Solid Edge part; units mm, degrees
sketch "Sketch1" plane through (0, 0, 0) normal (0, -1, 0) x (1, 0, 0)
  line L0 (-30, 0) -> (-5, 0)
  line L1 (-5, 0) -> (-5, -160)
  line L2 (-5, -160) -> (-20, -160)
  line L3 (-20, -160) -> (-20, -10)
  line L4 (-20, -10) -> (-30, -10)
  line L5 (-30, -10) -> (-30, 0)
  dimension "D1" = 30
  dimension "D2" = 20
revolve "RevolvedProtrusion1" add sketch "Sketch1" angle 360 about axis through (0, 0, 54) along (0, 0, -1)
sketch "Sketch2" plane through (0, 0, -160) normal (0, 0, -1) x (0, 1, 0)
  circle A0 centre (0, 0) radius 10
  circle A1 centre (0, 0) radius 20
extrude "Cutout1" cut sketch "Sketch2" against normal blind 20
cosmetic_thread "Thread1"
sketch "Sketch3" plane through (0, 0, 0) normal (0, 0, 1) x (1, 0, 0)
  circle A0 centre (0, 0) radius 30
  circle A1 centre (0, 0) radius 5
extrude "Ausprägung_1" add sketch "Sketch3" along normal blind 30
sketch "Sketch4" plane through (0, 0, 0) normal (0, 0, 1) x (1, 0, 0)
  line L0 (-61, 50) -> (-11, 50)
  line L1 (-11, 50) -> (-11, -50)
  line L2 (-11, -50) -> (-61, -50)
  line L3 (-61, -50) -> (-61, 50)
extrude "Cutout2" cut sketch "Sketch4" along normal up to next
mirror "Mirror1" about plane through (0, 0, 0) normal (1, 0, 0) of "Cutout2"
hole "Bohrung_1" at (11, -20, 15) direction (-1, 0, 0) diameter 10 end through all
hole "Hole1" at (11, 20, 15) direction (-1, 0, 0) diameter 10 end through all
extrude "Cutout4" [suppressed]
chamfer "Fase_2" distance 1 angle 45 2 edges at (0, -20, -140) (0, -10, -160)
chamfer "Fase_3" distance 1 angle 45 2 edges at (-5, 0, 30) (5, 0, -160)
properties material "Stahl"
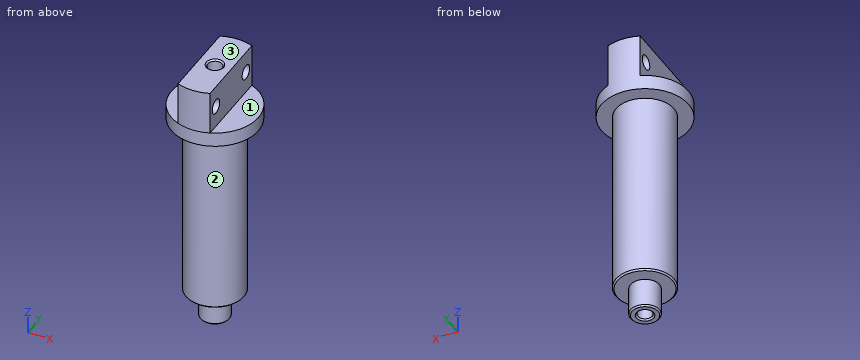
Could you check a few things on this model? Use its own coordinates, in mm. Face numbers are marked on the shaded views. A direction names the side the tool comes from. Give positions to 0.01 mm unless a question says otherwise; leave off trailing zeros. Loops run counter-clockwise (first coordinate to the right, second up) from the corner with the lowest first, then second, coordinate; pieces in that order, holes last. Notation, with made-up numbers: (78.25, 49) -> (93.25, 49) arc R20 ccw to (93.25, 53) -> close; hole circle Ø1 at (70.25, 71.25). An arc over 180 degrees is marked (long way). Return JSON: item names as keys, results as strings.
Item 1: If we section it at B-B on z = 15: List the corners of the cut face in (x, y) for me, plus the area to 3 significant figures.
Geometry results:
{"outline": "(-11, -27.91) arc R30 ccw to (11, -27.91) -> (11, -25) -> (-11, -25) -> close; (-11, -15) -> (11, -15) -> (11, 15) -> (-11, 15) -> close; (-11, 25) -> (11, 25) -> (11, 27.91) arc R30 ccw to (-11, 27.91) -> close; hole circle Ø10 at (0, 0)", "area": "771 mm²"}
Item 2: Which directions (+Z, -Z, +X, -X, +Y, -Y) give clear straight access to the entire face, cutting with the end or side of a thin tool? Please do the marked faces 1, 2 and 3.
Geometry results:
{"face 1": "+Z, +X, +Y, -Y", "face 2": "-Z", "face 3": "+Z, +X, -X, +Y, -Y"}
Item 3: If we section it at C-C on y = 0: List the corners of the cut face in (x, z) for me, plus the area to 3 significant figures.
Geometry results:
{"outline": "(-30, -10) -> (-20, -10) -> (-20, -139) -> (-19, -140) -> (-10, -140) -> (-10, -159) -> (-9, -160) -> (-6, -160) -> (-5, -159) -> (-5, 29) -> (-6, 30) -> (-11, 30) -> (-11, 0) -> (-30, 0) -> close; (5, -159) -> (6, -160) -> (9, -160) -> (10, -159) -> (10, -140) -> (19, -140) -> (20, -139) -> (20, -10) -> (30, -10) -> (30, 0) -> (11, 0) -> (11, 30) -> (6, 30) -> (5, 29) -> close", "area": "4,960 mm²"}
Item 4: I need wall thicknesses on L1, parallel to Z at x = 4, y = 20; L2, parallel to Y at x = 0, z = -116; L3, parallel to Y at x = -3.25, z = 15. Which ranges of each line are inside material? Lowest first, please. Write a range as from..to.
Geometry results:
{"L1": "z = -10..10, 20..30", "L2": "y = -20..-5, 5..20", "L3": "y = -29.82..-25, -15..-3.8, 3.8..15, 25..29.82"}
Item 5: I'm going to push flat-ended pins straight in: pin 1 (12 mm diameter, centred on x = 9.5, z = -122.5, fed in from +Y); pin 2 (11.5 mm diameter, centred on x = 0, y = 0, fed in from +Z); pin 3 (6 mm diameter, centred on x = 12.5, z = -88, fed in from -Y). Where does each tip first touch, or does it pass through?
Geometry results:
{"pin 1": "stops at y = 19.69", "pin 2": "stops at z = 29.75", "pin 3": "stops at y = -17.6"}
Item 6: If we section it at D-D on z = -68.5: List the corners of the cut face in (x, y) for me, plus the area to 3 significant figures.
Geometry results:
{"outline": "circle Ø40 at (0, 0); hole circle Ø10 at (0, 0)", "area": "1,180 mm²"}
Item 7: If we section it at A-A on x = 0: List the corners of the cut face in (y, z) for me.
Geometry results:
{"outline": "(-30, -10) -> (-20, -10) -> (-20, -139) -> (-19, -140) -> (-10, -140) -> (-10, -159) -> (-9, -160) -> (-6, -160) -> (-5, -159) -> (-5, 29) -> (-6, 30) -> (-30, 30) -> close; (5, -159) -> (6, -160) -> (9, -160) -> (10, -159) -> (10, -140) -> (19, -140) -> (20, -139) -> (20, -10) -> (30, -10) -> (30, 30) -> (6, 30) -> (5, 29) -> close; hole circle Ø10 at (-20, 15); hole circle Ø10 at (20, 15)"}
